Model file for the job. Use its own axes, mm. A direction names the side the tool comes from. Coordinates: 2 decimals unless noted, no trailing zeros. Order: outer loops, then holes, each group sorted by start corner. A loop starts at its lowest first (then second) coordinate and runs counter-clockwise, first axis right, second up. Notation, with made-up numbers: (19, 76) -> (63, 76) arc R34 ccw to (63, 111) -> close; hole circle Ø5 at (-14.75, -22). An arc over 180 degrees is marked (long way). Write item = value, one per line. Start each with the question number.
Q1. Wall check: line 1 (Z direction, x = -19.4, y = -10); line 2 (Z direction, x = -9, y = -181.5). Give the ranges that are in metal, low to high. Write a range as from..to.
Q2. Mould opens along X. For faces 1 (the face through (-19, 0, 0)), 2 (the face through (20, -228, -5)), 3 (the face through (18, -228, -4)) say: +X half, -X half, draft (parallel to the pull), parting line (faces both ways), or undercut.
Q3. Cut at A-A, the plane y = -345. List the corners of the cut face in (x, z), plus the area to 3 significant figures.
Q4. 3-axis set-ups, long thin cutter, end or side, ignore diameter. For faces 4 (the face through (19, -60, 0)), 5 (the face through (0, -197, -20)), 6 (the face through (0, -197, 18)): which of +Z, -Z, +X, -X, +Y, -Y reach the whole face in a straight line?
Q5. Flat gauge pins, fed straight in: pin 1 (12 mm diameter, centred on x = 1.5, z = 13.5, fed in from +Y); pin 2 (0.6 mm diameter, centred on y = -40, z = 19, fed in from +X); pin 3 (6.5 mm diameter, centred on y = -10, z = 14, fed in from +X). Where does each tip first touch, or does it go through?
Q6. Cut at D-D, the plane y = -244. List the corners of the cut face in (x, z).
Q7. Cut at B-B, the plane x = 11. List the corners of the cut face in (y, z), plus the area to 3 significant figures.
Q8. Cut at C-C, the plane y = -40. List the corners of the cut face in (x, z), plus the area to 3 significant figures.
from build123d import *

# Parameters (mm, degrees)
F0_W     = 40
F0_H     = 40
F0_W_2   = 36
F0_H_2   = 36
F1_DEPTH = 400
F2_W     = 220
F2_H     = 6
F3_DEPTH = 2
F5_DEPTH = 60
F6_R     = 2.5
F7_DEPTH = 25


with BuildPart() as f1:
    # F0 (on Front) → F1 (new body)
    with BuildSketch(Plane.XZ):
        Rectangle(F0_W, F0_H)
        Rectangle(F0_W_2, F0_H_2, mode=Mode.SUBTRACT)
    extrude(amount=F1_DEPTH)

    # F2 (on face) → F3 (cut)
    with BuildSketch(Plane.YZ.offset(20)):
        with Locations((-230, 0)):
            Rectangle(F2_W, F2_H)
    extrude(amount=-F3_DEPTH, mode=Mode.SUBTRACT)

    # F4 (on Front) → F5 (cut)
    with BuildSketch(Plane.XZ):
        Polygon((-5, -18), (-5, -20), (20, -20), (20, 20), (-5, 20), (-5, 18), (18, 18), (18, -18), align=None)
    extrude(amount=F5_DEPTH, mode=Mode.SUBTRACT)

    # F6 (on face) → F7 (cut)
    with BuildSketch(Plane(origin=(-20, 0, 0), x_dir=(0, -1, 0), z_dir=(-1, 0, 0))):
        with Locations((10, 14)):
            Circle(F6_R)
        with Locations((10, -14)):
            Circle(F6_R)
        with Locations((390, 14)):
            Circle(F6_R)
        with Locations((390, -14)):
            Circle(F6_R)
    extrude(amount=-F7_DEPTH, mode=Mode.SUBTRACT)


solid = f1.part
Here are the results:
q1.line_1 = -20..-16.5, -11.5..11.5, 16.5..20
q1.line_2 = -20..-18, 18..20
q2.face_1 = draft
q2.face_2 = +X half
q2.face_3 = undercut
q3.outline = (-20, -20) -> (20, -20) -> (20, 20) -> (-20, 20) -> close; hole (-18, -18) -> (18, -18) -> (18, 18) -> (-18, 18) -> close
q3.area = 304 mm²
q4.face_4 = +Z, -Z, +X, +Y
q4.face_5 = -Z, +X, -X, +Y, -Y
q4.face_6 = +Y, -Y
q5.pin_1 = -60
q5.pin_2 = -5
q5.pin_3 = -18
q6.outline = (-20, -20) -> (20, -20) -> (20, -3) -> (18, -3) -> (18, -18) -> (-18, -18) -> (-18, 18) -> (18, 18) -> (18, 3) -> (20, 3) -> (20, 20) -> (-20, 20) -> close
q7.outline = (-400, -20) -> (-60, -20) -> (-60, -18) -> (-400, -18) -> close; (-400, 18) -> (-60, 18) -> (-60, 20) -> (-400, 20) -> close
q7.area = 1,360 mm²
q8.outline = (-20, -20) -> (-5, -20) -> (-5, -18) -> (-18, -18) -> (-18, 18) -> (-5, 18) -> (-5, 20) -> (-20, 20) -> close
q8.area = 132 mm²
